Geometry: final body of the model. Coordinates: model frame, mm. A direction names the side the tool comes from. Coordinates: 2 decimals unless noted, no trailing zeros. Loops run counter-clockwise (first coordinate to the right, second up) from the corner with the lowest first, then second, coordinate; pieces in that order, holes last. Notation, with made-up numbers: (79.25, 68.25) - (131.25, 68.25) arc R25 ccw to (131.25, 99.25) - close; hole circle Ø10 at (15.25, -18). An arc over 180 degrees is marked (long way). Return JSON: item names as keys, results as strings.
Autodesk Inventor part; units mm, degrees
ref_plane "YZ Plane" through (0, 0, 0) normal (1, 0, 0) x (0, 1, 0)
ref_plane "XZ Plane" through (0, 0, 0) normal (0, 1, 0) x (-1, 0, 0)
ref_plane "XY Plane" through (0, 0, 0) normal (0, 0, 1) x (1, 0, 0)
sketch "Esquisse1" plane through (0, 0, 0) normal (0, 0, 1) x (1, 0, 0)
  line L0 (-151.6254, 54.2183) -> (148.3746, 54.2183)
  line L1 (148.3746, 54.2183) -> (148.3746, -10.7817)
  line L2 (148.3746, -10.7817) -> (-151.6254, -10.7817)
  line L3 (-151.6254, -10.7817) -> (-151.6254, 54.2183)
  point P0 (0, 0)
  dimension "d0" = 300
  dimension "d1" = 65
extrude "Extrusion1" add sketch "Esquisse1" along normal blind 4
sketch "Esquisse2" plane through (0, 0, 4) normal (0, 0, 1) x (1, 0, 0)
  line L0 (-141.6254, 49.2183) -> (138.3746, 49.2183)
  line L1 (138.3746, 49.2183) -> (138.3746, 39.2183)
  line L2 (138.3746, 39.2183) -> (-141.6254, 39.2183)
  line L3 (-141.6254, 39.2183) -> (-141.6254, 49.2183)
  line L4 (-141.6254, 34.2183) -> (138.3746, 34.2183)
  line L5 (138.3746, 34.2183) -> (138.3746, 24.2183)
  line L6 (138.3746, 24.2183) -> (-141.6254, 24.2183)
  line L7 (-141.6254, 24.2183) -> (-141.6254, 34.2183)
  line L8 (-141.6254, 19.2183) -> (138.3746, 19.2183)
  line L9 (138.3746, 19.2183) -> (138.3746, 9.2183)
  line L10 (138.3746, 9.2183) -> (-141.6254, 9.2183)
  line L11 (-141.6254, 9.2183) -> (-141.6254, 19.2183)
  line L12 (-141.6254, 4.2183) -> (138.3746, 4.2183)
  line L13 (138.3746, 4.2183) -> (138.3746, -5.7817)
  line L14 (138.3746, -5.7817) -> (-141.6254, -5.7817)
  line L15 (-141.6254, -5.7817) -> (-141.6254, 4.2183)
  line L16 (148.3746, 54.2183) -> (-151.6254, 54.2183)
  line L17 (148.3746, -10.7817) -> (148.3746, 54.2183)
  point P0 (0, 0)
  dimension "d4" = 5
  dimension "d5" = 10
  dimension "d6" = 5
  dimension "d7" = 10
  dimension "d8" = 5
  dimension "d9" = 10
  dimension "d10" = 5
  dimension "d11" = 10
  dimension "d12" = 280
  dimension "d13" = 10
extrude "Extrusion2" cut sketch "Esquisse2" against normal blind 1
Item 1: Section query A-A, the plane x = 4. Return loops of the section in (y, z).
Worked out:
{"outline": "(-10.78, 0) - (54.22, 0) - (54.22, 4) - (49.22, 4) - (49.22, 3) - (39.22, 3) - (39.22, 4) - (34.22, 4) - (34.22, 3) - (24.22, 3) - (24.22, 4) - (19.22, 4) - (19.22, 3) - (9.22, 3) - (9.22, 4) - (4.22, 4) - (4.22, 3) - (-5.78, 3) - (-5.78, 4) - (-10.78, 4) - close"}
Item 2: Section query B-B, the plane y = 28. Return loops of the section in (x, z).
Worked out:
{"outline": "(-151.63, 0) - (148.37, 0) - (148.37, 4) - (138.37, 4) - (138.37, 3) - (-141.63, 3) - (-141.63, 4) - (-151.63, 4) - close"}
Item 3: Reachability of faces 3 (the face through (-4, 22, 4)), 4 (the face through (-4, 14, 3)) from +Z, -Z, +X, -X, +Y, -Y: full face, straight path, thin tool, end or side. Return the list, or none.
Worked out:
{"face 3": "+Z, +X, -X, +Y, -Y", "face 4": "+Z"}
Item 4: First-contact query: pin 1 Ø5 at (x, y) = (65.5, 14) entering from +Z. Flat tip, straight axial feed; report the tip coordinate or a pass-through.
Worked out:
{"pin 1": "z = 3"}
Item 5: Ray query, probe 1 along Y at (x, z) = (-133.5, 3.8); probe 2 along X at (y, z) = (26.5, 3.6); probe 3 along Z at (x, y) = (21, 0). Return the intervals inside material, ascending. Write a range as from..to.
Worked out:
{"probe 1": "-10.78..-5.78, 4.22..9.22, 19.22..24.22, 34.22..39.22, 49.22..54.22", "probe 2": "-151.63..-141.63, 138.37..148.37", "probe 3": "0..3"}
Item 6: Mould query, pull axis Y, two halves, no side actions, for faces 1 (the face through (-4, 22, 0)), 2 (the face through (-4, 29, 3)). Classes: +Y half, -Y half, draft (parallel to the pull), parting line (faces both ways), or undercut.
Worked out:
{"face 1": "draft", "face 2": "undercut"}
